Read the model definition and answer for the solid it produces. Units are mm, in the model's axes. Face numbers are marked on the shaded views. A direction names the side the tool comes from. Coordinates: 2 decimals unless noted, no trailing zeros. Order: outer loops, then holes, each group sorted by start corner. A loop starts at its lowest first (then second) coordinate and runs counter-clockwise, first axis right, second up.
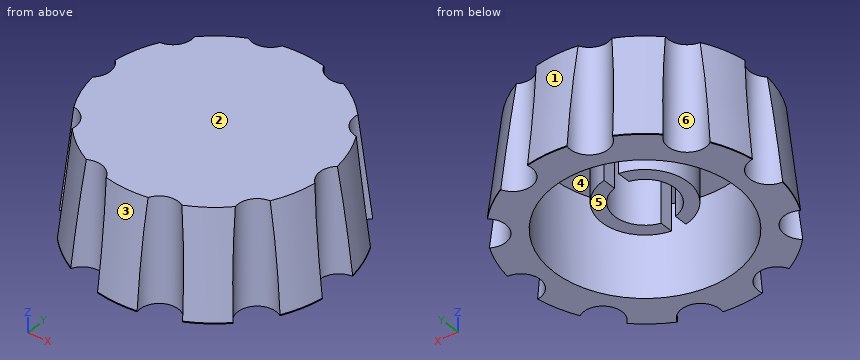
```python
from build123d import *

# Parameters (mm, degrees)
F0_R      = 13
F0_R_2    = 11.75
F0_R_3    = 3.15
F3_DEPTH  = 0.1
F3_FACE_R = 13
F2_R      = 11.75
F5_DEPTH  = 9.5
F6_R      = 2
F7_DEPTH  = 25
F8_DEPTH  = 11.0010001
F9_R      = 9.5
F10_DEPTH = 9.5
F11_DEPTH = 2.75


with BuildPart() as f3:
    # F0 (on Top) → F3 (new body)
    with BuildSketch(Plane.XY):
        Circle(F0_R)
        Circle(F0_R_2, mode=Mode.SUBTRACT)
        Circle(F0_R_2)
        Circle(F0_R_3, mode=Mode.SUBTRACT)
        Circle(F0_R_3)
    extrude(amount=F3_DEPTH)

    # F3_face (on face) → F4 section 0
    with BuildSketch(Plane.XY.offset(0.1)):
        Circle(F3_FACE_R)
    # F2 (on offset) → F4 section 1
    with BuildSketch(Plane.XY.offset(11)):
        Circle(F2_R)
    loft()

    # F0 (on Top) → F5 (cut)
    with BuildSketch(Plane.XY):
        Circle(F0_R_3)
    extrude(amount=F5_DEPTH, mode=Mode.SUBTRACT)

    # F6 (on face) → F7 (cut)
    with BuildSketch(Plane.XY.offset(11)):
        with Locations((13, 0)):
            Circle(F6_R)
        with Locations((10.5172209269, 7.6412082798)):
            Circle(F6_R)
        with Locations((4.0172209269, 12.3637347118)):
            Circle(F6_R)
        with Locations((-4.0172209269, 12.3637347118)):
            Circle(F6_R)
        with Locations((-10.5172209269, 7.6412082798)):
            Circle(F6_R)
        with Locations((-13, 0)):
            Circle(F6_R)
        with Locations((-10.5172209269, -7.6412082798)):
            Circle(F6_R)
        with Locations((-4.0172209269, -12.3637347118)):
            Circle(F6_R)
        with Locations((4.0172209269, -12.3637347118)):
            Circle(F6_R)
        with Locations((10.5172209269, -7.6412082798)):
            Circle(F6_R)
    extrude(amount=-F7_DEPTH, mode=Mode.SUBTRACT)

    # F6 (on face) → F8 (cut, through all)
    with BuildSketch(Plane.XY.offset(11)):
        with Locations((13, 0)):
            Circle(F6_R)
        with Locations((10.5172209269, 7.6412082798)):
            Circle(F6_R)
        with Locations((4.0172209269, 12.3637347118)):
            Circle(F6_R)
        with Locations((-4.0172209269, 12.3637347118)):
            Circle(F6_R)
        with Locations((-10.5172209269, 7.6412082798)):
            Circle(F6_R)
        with Locations((-13, 0)):
            Circle(F6_R)
        with Locations((-10.5172209269, -7.6412082798)):
            Circle(F6_R)
        with Locations((-4.0172209269, -12.3637347118)):
            Circle(F6_R)
        with Locations((4.0172209269, -12.3637347118)):
            Circle(F6_R)
        with Locations((10.5172209269, -7.6412082798)):
            Circle(F6_R)
    extrude(amount=-F8_DEPTH, mode=Mode.SUBTRACT)

    # F9 (on face) → F10 (cut)
    with BuildSketch(Plane(origin=(0, 0, 0), x_dir=(1, 0, 0), z_dir=(0, 0, -1))):
        Circle(F9_R)
        with BuildLine():
            ThreePointArc((0.75, 4.4370598373), (4.5, 0), (0.75, -4.4370598373))
            Line((0.75, -4.4370598373), (0.75, -3.0594117082))
            ThreePointArc((0.75, -3.0594117082), (0, -3.15), (-0.75, -3.0594117082))
            Line((-0.75, -3.0594117082), (-0.75, -4.4370598373))
            ThreePointArc((-0.75, -4.4370598373), (-4.5, 0), (-0.75, 4.4370598373))
            Line((-0.75, 4.4370598373), (-0.75, 3.0594117082))
            ThreePointArc((-0.75, 3.0594117082), (0, 3.15), (0.75, 3.0594117082))
            Line((0.75, 3.0594117082), (0.75, 4.4370598373))
        make_face(mode=Mode.SUBTRACT)
    extrude(amount=-F10_DEPTH, mode=Mode.SUBTRACT)

    # F11 (cut): faces of the model
    f11_faces = [f3.faces().sort_by_distance(p)[0] for p in [
        (-3.2463392443, 0, 0),
        (0.8463392443, 3.7482357727, 0),
    ]]
    extrude(f11_faces, amount=-F11_DEPTH, mode=Mode.SUBTRACT)


solid = f3.part
```
1) A cutting plane is placed at C-C, the plane x = 0. Determine the outline of the cut face in (y, z).
A:
outline: (-13, 0) - (-9.5, 0) - (-9.5, 9.5) - (9.5, 9.5) - (9.5, 0) - (13, 0) - (13, 0.1) - (11.75, 11) - (-11.75, 11) - (-13, 0.1) - close
2) Which of the six approach directions +Z, -Z, +X, -X, +Y, -Y give full straight-line access (tool end or side, diameter ignored) to the marked faces 5 and 6?
A:
face 5: -Z
face 6: +Z, -Z
3) A cutting plane is placed at D-D, the plane z = 1. Determine the outline of the cut face in (x, y), and give its area (3 significant figures).
A:
outline: (-12.74, -1.98) arc R12.9 ccw to (-11.48, -5.89) arc R2 cw to (-9.14, -9.1) arc R12.9 ccw to (-5.82, -11.51) arc R2 cw to (-2.05, -12.73) arc R12.9 ccw to (2.05, -12.73) arc R2 cw to (5.82, -11.51) arc R12.9 ccw to (9.14, -9.1) arc R2 cw to (11.48, -5.89) arc R12.9 ccw to (12.74, -1.98) arc R2 cw to (12.74, 1.98) arc R12.9 ccw to (11.48, 5.89) arc R2 cw to (9.14, 9.1) arc R12.9 ccw to (5.82, 11.51) arc R2 cw to (2.05, 12.73) arc R12.9 ccw to (-2.05, 12.73) arc R2 cw to (-5.82, 11.51) arc R12.9 ccw to (-9.14, 9.1) arc R2 cw to (-11.48, 5.89) arc R12.9 ccw to (-12.74, 1.98) arc R2 cw to start; hole circle Ø19 at (0, 0)
area: 182 mm2
4) Determine the mould class of the marked faces 1, 2, 3 and 4 for opening direction Y: pulls with the +Y half, pulls with the -Y half, needs draft (parallel to the pull), parting line crosses it, or undercut.
A:
face 1: pulls with the +Y half
face 2: needs draft
face 3: pulls with the -Y half
face 4: undercut
5) Flat-ended cylindrical pins translate along their axes: pin 1 Ø5 at (x, z) = (-7, 9) entering from -Y; pin 2 Ø4 at (x, y) = (-2, 1) entering from -Z; pin 3 Ø1.1 at (y, z) = (-4, 5.5) entering from -X; pin 4 Ø15 at (x, y) = (4, 0.5) entering from -Z. Find the tip coordinate at first contact, or state that the pin passes through.
A:
pin 1: stops at y = -10.93
pin 2: stops at z = 2.75
pin 3: stops at x = -11.9
pin 4: stops at z = 0
6) Straight lines are drawn through the part: line 1 (X direction, y = 3.25, z = 9); line 2 (Y direction, x = 3.5, z = 5); line 3 (Z direction, x = -6, y = 4.25). For each, find the intervals that lie inside material, in ascending order.
A:
line 1: x = -11.53 to -8.93, -3.11 to -0.75, 0.75 to 3.11, 8.93 to 11.53
line 2: y = -10.43 to -8.83, -2.83 to 2.83, 8.83 to 10.43
line 3: z = 9.5 to 11
7) A cutting plane is placed at A-A, the plane z = 6. State how many separate pieces and enclosed holes the cut face has, and give its area (3 significant figures).
A:
separate pieces: 3
enclosed holes: 1
area: 187 mm2
8) A cutting plane is placed at B-B, the plane y = 0. Determine the outline of the cut face in (x, z).
A:
outline: (-11, 0) - (-9.5, 0) - (-9.5, 9.5) - (-4.5, 9.5) - (-4.5, 2.75) - (-3.15, 2.75) - (-3.15, 9.5) - (3.15, 9.5) - (3.15, 2.75) - (4.5, 2.75) - (4.5, 9.5) - (9.5, 9.5) - (9.5, 0) - (11, 0) - (11, 11) - (-11, 11) - close
